Here's how the part is built. I have some questions about the finished solid (model axes, mm). Round coordinates to 2 decimals unless told otherwise and drop trailing zeros. Loops run counter-clockwise (first coordinate to the right, second up) from the corner with the lowest first, then second, coordinate; pieces in that order, holes last. Notation, with made-up numbers: M 42.25,22 L 57.25,22 A20 cw 57.25,56 Z; hole C 13,-37 d6. An arc over 180 degrees is marked long. Use a Markdown table: item, result.
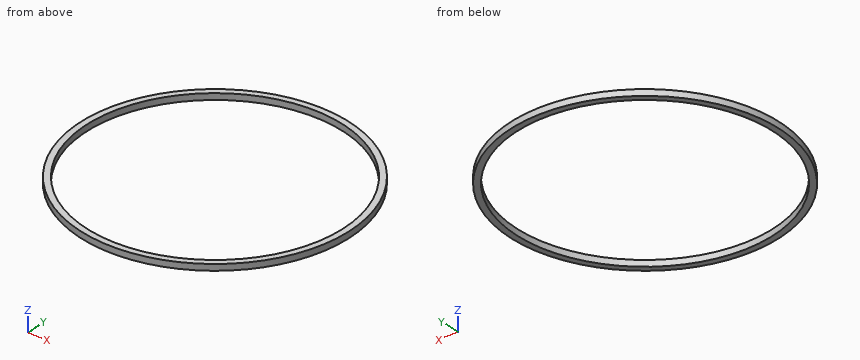
from build123d import *

# Parameters (mm, degrees)
F1_W     = 180
F1_H     = 180
F1_W_2   = 179.4
F1_H_2   = 179.4
F2_DEPTH = 0.3
F1_W_3   = 129.7133469
F1_H_3   = 140
F1_W_4   = 129.1133469
F1_H_4   = 139.4
F1_R     = 6.5
F1_R_2   = 6.2
F1_W_5   = 80
F1_H_5   = 80


with BuildPart() as f2:
    # F1 (on Top) → F2 (new body)
    with BuildSketch(Plane.XY):
        with Locations((-1.4824382961, 17.8632308638)):
            Rectangle(F1_W, F1_H)
        with Locations((-1.4824382961, 17.8632308638)):
            Rectangle(F1_W_2, F1_H_2, mode=Mode.SUBTRACT)
    extrude(amount=F2_DEPTH)


with BuildPart() as f2b:
    # F1 (on Top) → F2, piece 2 (new body)
    with BuildSketch(Plane.XY):
        Polygon((-81.3541731706, 97.8632308638), (-81.4824382961, 97.8632308638), (-81.4824382961, 95.4210562907), (-81.1824382961, 95.666005265), (-81.1824382961, 97.5632308638), (-79.8844793249, 97.5632308638), align=None)
        Polygon((-79.8541731706, 97.8632308638), (-81.3541731706, 97.8632308638), (-79.8844793249, 97.5632308638), (-78.3844793249, 97.5632308638), align=None)
        Polygon((68.2309086039, 97.8632308638), (-79.8541731706, 97.8632308638), (-78.3844793249, 97.5632308638), (67.9309086039, 97.5632308638), (67.9309086039, -61.8367691362), (-81.1824382961, -61.8367691362), (-81.1824382961, 95.2787069303), (-81.4824382961, 95.0337579561), (-81.4824382961, -62.1367691362), (68.2309086039, -62.1367691362), align=None)
        Polygon((-87.8824382961, 99.1958074024), (-81.3541731706, 97.8632308638), (-79.8541731706, 97.8632308638), (-88.1824382961, 99.5632308638), (-88.1824382961, 89.5632308638), (-81.4824382961, 95.0337579561), (-81.4824382961, 95.4210562907), (-87.8824382961, 90.1954781727), align=None)
    extrude(amount=F2_DEPTH)


with BuildPart() as f2c:
    # F1 (on Top) → F2, piece 3 (new body)
    with BuildSketch(Plane.XY):
        with Locations((-6.6257648461, 17.8632308638)):
            Rectangle(F1_W_3, F1_H_3)
        with Locations((-6.6257648461, 17.8632308638)):
            Rectangle(F1_W_4, F1_H_4, mode=Mode.SUBTRACT)
    extrude(amount=F2_DEPTH)


with BuildPart() as f2d:
    # F1 (on Top) → F2, piece 4 (new body)
    with BuildSketch(Plane.XY):
        with Locations((78.3742351539, -51.8367691362)):
            Circle(F1_R)
        with Locations((78.3742351539, -51.8367691362)):
            Circle(F1_R_2, mode=Mode.SUBTRACT)
    extrude(amount=F2_DEPTH)


with BuildPart() as f2e:
    # F1 (on Top) → F2, piece 5 (new body)
    with BuildSketch(Plane.XY):
        with Locations((-1.4824382961, 17.8632308638)):
            Rectangle(F1_W_5, F1_H_5)
    extrude(amount=F2_DEPTH)


solid = f2d.part
1. Imagine slicing it at A-A, the plane x = 83.5. Write out the boundary of the cut face in (y, z), then the cut area to 3 significant figures.
Answer sheet:
| item | result |
|---|---|
| outline | M -55.83,0 L -55.32,0 L -55.32,0.3 L -55.83,0.3 Z; M -48.35,0 L -47.84,0 L -47.84,0.3 L -48.35,0.3 Z |
| area | 0.305 mm2 |
2. Imagine slicing it at B-B, the plane y = -49.25. Write out the boundary of the cut face in (x, z), then the cut area to 3 significant figures.
Answer sheet:
| item | result |
|---|---|
| outline | M 72.41,0 L 72.74,0 L 72.74,0.3 L 72.41,0.3 Z; M 84.01,0 L 84.34,0 L 84.34,0.3 L 84.01,0.3 Z |
| area | 0.197 mm2 |
3. Imagine slicing it at C-C, the plane z = 0.15. Write out the boundary of the cut face in (x, y), then the cut area to 3 significant figures.
Answer sheet:
| item | result |
|---|---|
| outline | C 78.37,-51.84 d13; hole C 78.37,-51.84 d12.4 |
| area | 12.0 mm2 |
4. For pin 1 Ø2 at (x, y) = (82, -49.5) entering from +Z, with a flat end and sliding along its axis, tell me the tip position at first contact or that it passes through.
Answer sheet:
| item | result |
|---|---|
| pin 1 | through |
5. I need wall thicknesses on probe 1 along X at (y, z) = (-53.5, 0.25); probe 2 along Y at (x, z) = (75.5, 0.25); probe 3 along Y at (x, z) = (81, 0.2). Which ranges of each line are inside material? Lowest first, please. Write a range as from..to.
Answer sheet:
| item | result |
|---|---|
| probe 1 | 72.09..72.4, 84.35..84.66 |
| probe 2 | -57.67..-57.33, -46.34..-46.01 |
| probe 3 | -57.78..-57.45, -46.22..-45.89 |
